Check sheet for the drawn part. Datum: minimum x, y, z corner. Units: mm. Give positions to 0.01 mm unless a question says otherwise; leave off trailing zeros. Loops run counter-clockwise (first coordinate to the right, second up) from the corner with the lowest first, then second, coordinate; pieces in that order, holes last. Notation, with made-up numbers: (-5.5, 53.5) - (9.5, 53.5) arc R11 cw to (9.5, 66.5) - close; hole circle Ø2 at (66.25, -10.75). An arc over 180 degrees is marked (long way). Use a Markdown table: item, result. Add a question column.
1. Cross-section at A-A on z = 3.74. Enter the section's corners in (x, y), and give its area (3 significant figures).
2. Cross-section at B-B on x = 7. Enter the section's corners in (y, z).
3. Cross-section at C-C on y = 0.4. Enter the section's corners in (x, z).
4. Cross-section at D-D on x = 31.5. Enter the section's corners in (y, z).
5. Depth check by flat-ended pin: P1, Ø10, axis at x = 14, z = 9, coming from the -Y side; P2, Ø3, axis at x = 15, z = 38.74, coming from the +Y side; P3, Ø0.5, axis at x = 8.5, y = 0.5, coming from the +Z side; P4, Ø0.5, axis at y = 0.5, z = 4.5, coming from the -X side. Enter the tip coordinate at first touch or a pass-through.
6. Material ranges on L1, parallel to Z at x = 15, y = 0.45; L2, parallel to X at y = 0.9, z = 21; L3, parallel to X at y = 0.55, z = 3.74, recorded low to high.
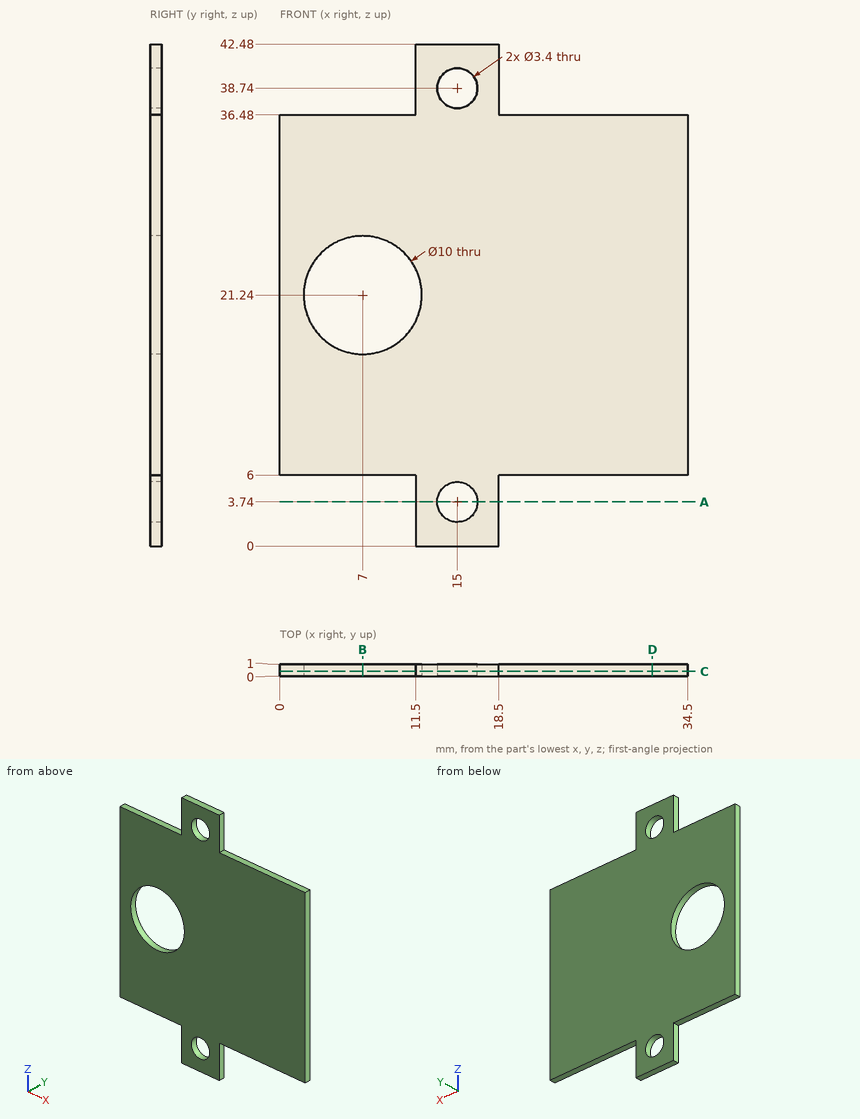
Values found:
| question | item | result |
|---|---|---|
| 1 | outline | (11.5, 0) - (13.3, 0) - (13.3, 1) - (11.5, 1) - close; (16.7, 0) - (18.5, 0) - (18.5, 1) - (16.7, 1) - close |
| 1 | area | 3.60 mm2 |
| 2 | outline | (0, 6) - (1, 6) - (1, 16.24) - (0, 16.24) - close; (0, 26.24) - (1, 26.24) - (1, 36.48) - (0, 36.48) - close |
| 3 | outline | (0, 6) - (11.5, 6) - (11.5, 0) - (18.5, 0) - (18.5, 6) - (34.5, 6) - (34.5, 36.48) - (18.5, 36.48) - (18.5, 42.48) - (11.5, 42.48) - (11.5, 36.48) - (0, 36.48) - close; hole circle Ø10 at (7, 21.24); hole circle Ø3.4 at (15, 3.74); hole circle Ø3.4 at (15, 38.74) |
| 4 | outline | (0, 6) - (1, 6) - (1, 36.48) - (0, 36.48) - close |
| 5 | P1 | stops at y = 0 |
| 5 | P2 | passes through |
| 5 | P3 | stops at z = 36.48 |
| 5 | P4 | stops at x = 11.5 |
| 6 | L1 | z = 0 to 2.04, 5.44 to 37.04, 40.44 to 42.48 |
| 6 | L2 | x = 0 to 2.01, 11.99 to 34.5 |
| 6 | L3 | x = 11.5 to 13.3, 16.7 to 18.5 |
